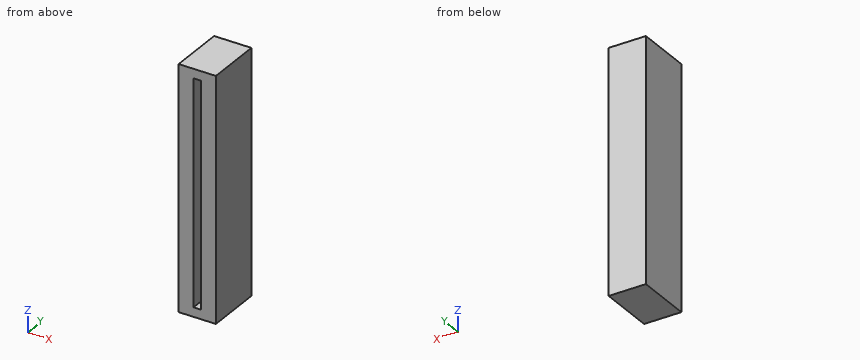
```python
from build123d import *

# Parameters (mm, degrees)
F0_W     = 10
F0_H     = 65
F1_DEPTH = 15
F2_W     = 2
F2_H     = 60
F3_DEPTH = 10


# Not quite as in the source:
# - a feature names something its author has since deleted; it is built from what else it names


with BuildPart() as f1:
    # F0 (on Front) → F1 (new body)
    with BuildSketch(Plane.XZ):
        Rectangle(F0_W, F0_H)
    extrude(amount=F1_DEPTH)

    # F2 (on face) → F3 (cut)
    with BuildSketch(Plane.XZ.offset(15)):
        Rectangle(F2_W, F2_H)
    extrude(amount=-F3_DEPTH, mode=Mode.SUBTRACT)


solid = f1.part
```
Geometry: final body of the model. Coordinates: model frame, mm. Round coordinates to 2 decimals unless told otherwise and drop trailing zeros. Loops run counter-clockwise (first coordinate to the right, second up) from the corner with the lowest first, then second, coordinate; pieces in that order, holes last. Notation, with made-up numbers: (25.5, 51) -> (74.5, 51) arc R21 cw to (74.5, 76) -> close; hole circle Ø11 at (22, 31). An arc over 180 degrees is marked (long way). Write each question's results on one line, items separated by ' | '.
Item 1: Cut plane C-C on x = 0. Return the cut outline in (y, z), and give its area (3 significant figures).
Answers below:
outline: (-15, -32.5) -> (0, -32.5) -> (0, 32.5) -> (-15, 32.5) -> (-15, 30) -> (-5, 30) -> (-5, -30) -> (-15, -30) -> close | area: 375 mm²
Item 2: Cut plane B-B on z = 16. Return the cut outline in (x, y).
Answers below:
outline: (-5, -15) -> (-1, -15) -> (-1, -5) -> (1, -5) -> (1, -15) -> (5, -15) -> (5, 0) -> (-5, 0) -> close
Item 3: Line query: probe 1 along X at (y, z) = (-14, 12); probe 2 along Y at (x, z) = (0, 25). Output: solid intervals per line, ascending. Write a range as [from, to].
Answers below:
probe 1: x = [-5, -1], [1, 5] | probe 2: y = [-5, 0]
Item 4: Cut plane A-A on y = -13.25. Return the cut outline in (x, z).
Answers below:
outline: (-5, -32.5) -> (5, -32.5) -> (5, 32.5) -> (-5, 32.5) -> close; hole (-1, -30) -> (1, -30) -> (1, 30) -> (-1, 30) -> close
